from build123d import *

# Parameters (mm, degrees)
F0_R     = 3.25
F1_DEPTH = 0.3
F2_R     = 5
F3_R     = 0.3
F4_W     = 22
F4_H     = 0.1
F5_DEPTH = 0.05


with BuildPart() as f1:
    # F0 (on Top) → F1 (new body)
    with BuildSketch(Plane.XY):
        with BuildLine():
            Line((13.2, 4.35), (-13.2, 4.35))
            add(Edge.make_bspline(
                [(-13.2, 4.35), (-23.9595582635, -1.9535795887), (-8.7692884448, -6.141299865)],
                knots=[2.4980915448, 2.4980915448, 2.4980915448, 4.1520515858, 4.1520515858, 4.1520515858], degree=2, weights=[1, 0.6771012168, 1]))
            ThreePointArc((-8.7692884448, -6.141299865), (-8.5065273892, -6.5651174574), (-8.6965923284, -7.0261381108))
            ThreePointArc((-8.6965923284, -7.0261381108), (-12.3142829071, -11.4828313169), (-9.8142494559, -16.65))
            ThreePointArc((-9.8142494559, -16.65), (-9.7441006003, -16.6877931911), (-9.6776213413, -16.7317214891))
            ThreePointArc((-9.6776213413, -16.7317214891), (-9.3154283119, -17.5296015758), (-9.8142494559, -18.25))
            ThreePointArc((-9.8142494559, -18.25), (-12.1461150395, -24.2628738838), (-7, -28.15))
            Line((-7, -28.15), (7, -28.15))
            ThreePointArc((7, -28.15), (12.1461150395, -24.2628738838), (9.8142494559, -18.25))
            ThreePointArc((9.8142494559, -18.25), (9.7441006003, -18.2122068089), (9.6776213413, -18.1682785109))
            ThreePointArc((9.6776213413, -18.1682785109), (9.3118539071, -17.45), (9.6776213413, -16.7317214891))
            ThreePointArc((9.6776213413, -16.7317214891), (9.7441006003, -16.6877931911), (9.8142494559, -16.65))
            ThreePointArc((9.8142494559, -16.65), (12.3142829071, -11.4828313169), (8.6965923284, -7.0261381108))
            ThreePointArc((8.6965923284, -7.0261381108), (8.5065273892, -6.5651174574), (8.7692884448, -6.141299865))
            add(Edge.make_bspline(
                [(8.7692884448, -6.141299865), (23.9595582635, -1.9535795887), (13.2, 4.35)],
                knots=[5.272726375, 5.272726375, 5.272726375, 6.926686416, 6.926686416, 6.926686416], degree=2, weights=[1, 0.6771012168, 1]))
        make_face()
        with Locations((-7, -22.8)):
            Circle(F0_R, mode=Mode.SUBTRACT)
        with Locations((-7, -12.1)):
            Circle(F0_R, mode=Mode.SUBTRACT)
        with Locations((7, -22.8)):
            Circle(F0_R, mode=Mode.SUBTRACT)
        with Locations((7, -12.1)):
            Circle(F0_R, mode=Mode.SUBTRACT)
        with BuildLine():
            ThreePointArc((-3.9615510182, -7.6965550094), (-4.0576261026, -7.3030225288), (-3.7319495204, -7.0621221367))
            add(Edge.make_bspline(
                [(-3.7319495204, -7.0621221367), (0, -7.4428760906), (3.7319495204, -7.0621221367)],
                knots=[4.4842359958, 4.4842359958, 4.4842359958, 4.9405419649, 4.9405419649, 4.9405419649], degree=2, weights=[1, 0.974085812, 1]))
            ThreePointArc((3.7319495204, -7.0621221367), (4.0576261026, -7.3030225288), (3.9615510182, -7.6965550094))
            ThreePointArc((3.9615510182, -7.6965550094), (1.6516765197, -12.233925164), (4.1857505441, -16.65))
            Line((4.1857505441, -16.65), (-4.1857505441, -16.65))
            ThreePointArc((-4.1857505441, -16.65), (-1.6516765197, -12.233925164), (-3.9615510182, -7.6965550094))
        make_face(mode=Mode.SUBTRACT)
    extrude(amount=F1_DEPTH)

    # F2
    f2_edges = [f1.edges().sort_by_distance(p)[0] for p in [
        (13.2, 4.35, 0.15),
        (-13.2, 4.35, 0.15),
    ]]
    fillet(f2_edges, radius=F2_R)

    # F3
    f3_edges = [f1.edges().sort_by_distance(p)[0] for p in [
        (-4.185751, -16.65, 0.15),
        (4.185751, -16.65, 0.15),
    ]]
    fillet(f3_edges, radius=F3_R)

    # F4 (on face) → F5 (cut)
    with BuildSketch(Plane(origin=(0, 0, 0), x_dir=(1, 0, 0), z_dir=(0, 0, -1))):
        with Locations((0, 17.45)):
            Rectangle(F4_W, F4_H)
    extrude(amount=-F5_DEPTH, mode=Mode.SUBTRACT)


solid = f1.part
Verification items for the finished model (mm, model axes). Give positions to 0.01 mm unless a question says otherwise; leave off trailing zeros. Order: outer loops, then holes, each group sorted by start corner. A loop starts at its lowest first (then second) coordinate and runs counter-clockwise, first axis right, second up. Notation, with made-up numbers: M 75,26 L 113,26 A11 cw 113,43 Z; hole C 27,44.25 d1. An arc over 180 degrees is marked long. Use one line per item in the form item = value. Start each with the question number.
Q1. Section check B-B (x = 6.5). Enter the section's corners in (y, z), then the cut area to 3 significant figures.
Q2. Section check C-C (y = -22.8). Enter the section's corners in (x, z).
Q3. Section check A-A (y = -12.1). Enter the section's corners in (x, z).
Q4. Section check D-D (x = -7.5). Enter the section's corners in (y, z).
Q5. Scan lines: line 1 along Y through (x, z) = (-7, 0.2); line 2 along Y through (x, z) = (0.5, 0.15). Record each from-to range of solid material in increasing order. Write a range as [from, to].
Evaluation:
q1.outline = M -28.15,0 L -26.01,0 L -26.01,0.3 L -28.15,0.3 Z; M -19.59,0 L -17.5,0 L -17.5,0.05 L -17.4,0.05 L -17.4,0 L -15.31,0 L -15.31,0.3 L -19.59,0.3 Z; M -8.89,0 L 4.35,0 L 4.35,0.3 L -8.89,0.3 Z
q1.area = 5.89 mm2
q2.outline = M -12.35,0 L -10.25,0 L -10.25,0.3 L -12.35,0.3 Z; M -3.75,0 L 3.75,0 L 3.75,0.3 L -3.75,0.3 Z; M 10.25,0 L 12.35,0 L 12.35,0.3 L 10.25,0.3 Z
q3.outline = M -12.35,0 L -10.25,0 L -10.25,0.3 L -12.35,0.3 Z; M -3.75,0 L -1.65,0 L -1.65,0.3 L -3.75,0.3 Z; M 1.65,0 L 3.75,0 L 3.75,0.3 L 1.65,0.3 Z; M 10.25,0 L 12.35,0 L 12.35,0.3 L 10.25,0.3 Z
q4.outline = M -28.13,0 L -26.01,0 L -26.01,0.3 L -28.13,0.3 Z; M -19.59,0 L -17.5,0 L -17.5,0.05 L -17.4,0.05 L -17.4,0 L -15.31,0 L -15.31,0.3 L -19.59,0.3 Z; M -8.89,0 L 4.35,0 L 4.35,0.3 L -8.89,0.3 Z
q5.line_1 = [-28.15, -26.05], [-19.55, -15.35], [-8.85, 4.35]
q5.line_2 = [-28.15, -16.65], [-7.25, 4.35]
